```python
from build123d import *

# Parameters (mm, degrees)
F0_R     = 50.8
F1_DEPTH = 304.8
F2_R     = 38.1
F3_DEPTH = 279.4
F4_R     = 9.525
F5_DEPTH = 38.1
F6_R     = 6.35
F7_DEPTH = 91.948


with BuildPart() as f1:
    # F0 (on Right) → F1 (new body)
    with BuildSketch(Plane.YZ):
        Circle(F0_R)
    extrude(amount=F1_DEPTH)

    # F2 (on face) → F3 (cut)
    with BuildSketch(Plane.YZ.offset(304.8)):
        Circle(F2_R)
    extrude(amount=-F3_DEPTH, mode=Mode.SUBTRACT)

    # F4 (on face) → F5 (join)
    with BuildSketch(Plane(origin=(0, 0, 0), x_dir=(0, -1, 0), z_dir=(-1, 0, 0))):
        Circle(F4_R)
    extrude(amount=F5_DEPTH)

    # F6 (on face) → F7 (cut)
    with BuildSketch(Plane(origin=(-38.1, 0, 0), x_dir=(0, -1, 0), z_dir=(-1, 0, 0))):
        Circle(F6_R)
    extrude(amount=-F7_DEPTH, mode=Mode.SUBTRACT)


solid = f1.part
```
The listing builds one solid part. Answer for the finished solid, in the listing's coordinates (mm). A direction names the side the tool comes from. Coordinates: 2 decimals unless noted, no trailing zeros. Write each loop counter-clockwise with the first axis right and the second up, starting at its lowest first coordinate (ties: lowest second). Pieces come first, ordered by that corner, then holes. Notation, with made-up numbers: (76, -36.5) - (103, -36.5) arc R25 ccw to (103, -3.5) - close; hole circle Ø7 at (3.5, 57). An arc over 180 degrees is marked (long way). Return JSON: item names as keys, results as strings. Group by question number.
1. A cutting plane is placed at C-C, the plane x = 154.5. Determine the outline of the cut face in (y, z).
2. Which of the six approach directions +Z, -Z, +X, -X, +Y, -Y give full straight-line access (tool end or side, diameter ignored) to faces 1 (the flat face through (-38.1, -2, -6.2)), 2 (the flat face through (25.4, 8, 1)), 3 (the cylindrical face through (-18.783, 7.559, -5.796))?
3. Straight lines are drawn through the part: L1, parallel to Z at x = 190, y = 0; L2, parallel to X at y = -11.5, z = -11.5; L3, parallel to X at y = -34, z = 23. For each, find the intervals that lie inside material, in ascending order.
4. A cutting plane is placed at D-D, the plane z = -18.5. Determine the outline of the cut face in (x, y), plus the area to 3 significant figures.
5. A cutting plane is placed at A-A, the plane z = 0. Determine the outline of the cut face in (x, y) (3 decimals), plus the area to 3 significant figures.
6. Determine the mould class of faces 4 (the cylindrical face through (167.056, -30.235, -23.183)), 5 (the cylindrical face through (-6.79, 1.38, -6.2)), 6 (the cylindrical face through (150.266, -11.012, -49.592)), 7 (the flat face through (304.8, 7, 38)) for opening direction Z: released by +Z, released by -Z, zero draft, split by the parting line, or undercut.
7. Given pin 1 (3 mm diameter, centred on x = 67, z = -14.5, fed in from -Y); pin 2 (10 mm diameter, centred on x = 31.5, y = 4, fed in from +Z); pin 3 (23 mm diameter, centred on y = -2, z = 13.5, fed in from +X); pin 4 (10 mm diameter, centred on y = 0, z = 0, fed in from -X), each flat-ended and moving along its own axis, determine where each tip first touches the part or whether it passes through.
Ans:
{
 "1": {"outline": "circle Ø101.6 at (0, 0); hole circle Ø76.2 at (0, 0)"},
 "2": {"face 1": "+Z, -Z, -X, +Y, -Y", "face 2": "+X", "face 3": "-X"},
 "3": {"L1": "-50.8 to -38.1, 38.1 to 50.8", "L2": "0 to 25.4", "L3": "0 to 304.8"},
 "4": {"outline": "(0, -47.31) - (304.8, -47.31) - (304.8, -33.31) - (25.4, -33.31) - (25.4, 33.31) - (304.8, 33.31) - (304.8, 47.31) - (0, 47.31) - close", "area": "10,200 mm²"},
 "5": {"outline": "(-38.1, -9.525) - (0, -9.525) - (0, -50.8) - (304.8, -50.8) - (304.8, -38.1) - (25.4, -38.1) - (25.4, -6.35) - (-38.1, -6.35) - close; (-38.1, 6.35) - (25.4, 6.35) - (25.4, 38.1) - (304.8, 38.1) - (304.8, 50.8) - (0, 50.8) - (0, 9.525) - (-38.1, 9.525) - close", "area": "9,600 mm²"},
 "6": {"face 4": "undercut", "face 5": "undercut", "face 6": "split by the parting line", "face 7": "zero draft"},
 "7": {"pin 1": "y = -49.11", "pin 2": "z = 50.8", "pin 3": "x = 25.4", "pin 4": "through"}
}
